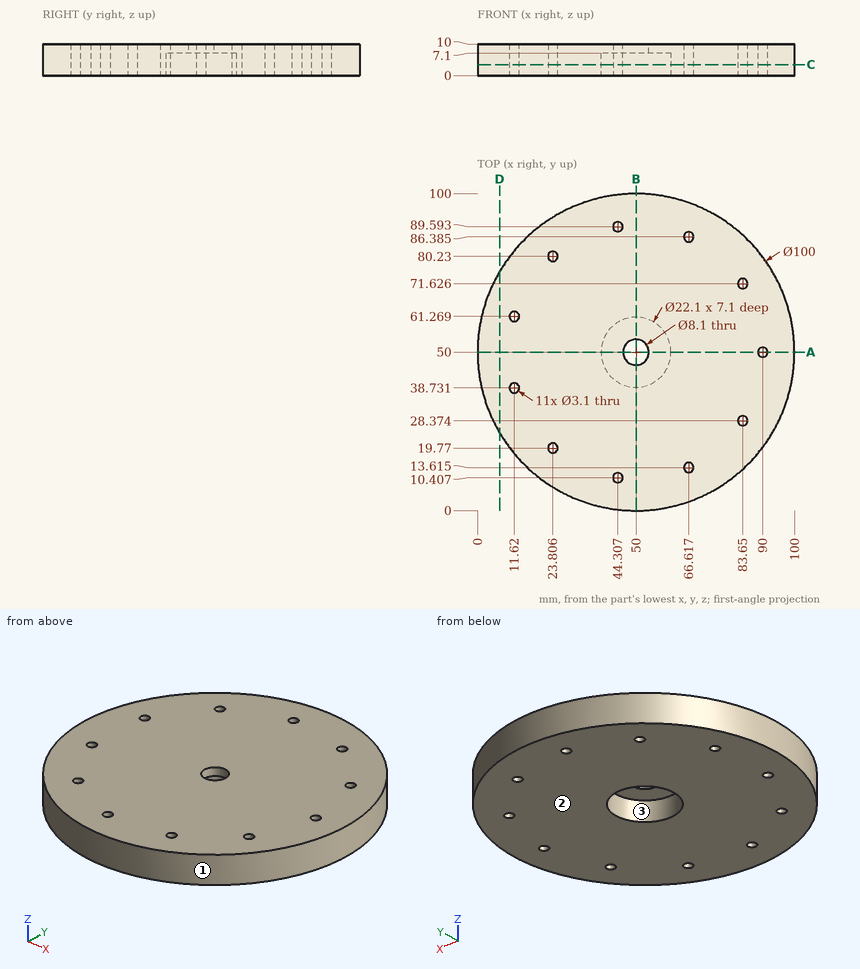
Source: three-view drawing plus pictorial views. Frame: mm from the lowest corner of the part. Round coordinates to 2 decimals unless told otherwise and drop trailing zeros. Order: outer loops, then holes, each group sorted by start corner. A loop starts at its lowest first (then second) coordinate and runs counter-clockwise, first axis right, second up. Notation, with made-up numbers: (66.5, 28) - (70.5, 28) arc R13 ccw to (70.5, 36) - close; hole circle Ø2 at (-18.75, 20.5). An arc over 180 degrees is marked (long way). Write each question's results on one line, items separated by ' | '.
Item 1: Section A-A, the plane y = 50. Return the cut outline in (x, z).
Completed:
outline: (0, 0) - (38.95, 0) - (38.95, 7.1) - (45.95, 7.1) - (45.95, 10) - (0, 10) - close; (54.05, 7.1) - (61.05, 7.1) - (61.05, 0) - (88.45, 0) - (88.45, 10) - (54.05, 10) - close; (91.55, 0) - (100, 0) - (100, 10) - (91.55, 10) - close
Item 2: Material intervals for line 1 along Y through (x, z) = (50, 7.9); line 2 along X through (y, z) = (14.5, 9) (1 decimal); line 3 along Y through (x, z) = (49, 1.25) (1 decimal), sorted ascending. Write a range as [from, to].
Completed:
line 1: [0, 45.95], [54.05, 100] | line 2: [14.8, 65.3], [67.9, 85.2] | line 3: [0, 39], [61, 100]
Item 3: Section B-B, the plane x = 50. Return the cut outline in (y, z).
Completed:
outline: (0, 0) - (38.95, 0) - (38.95, 7.1) - (45.95, 7.1) - (45.95, 10) - (0, 10) - close; (54.05, 7.1) - (61.05, 7.1) - (61.05, 0) - (100, 0) - (100, 10) - (54.05, 10) - close
Item 4: Section C-C, the plane z = 3.5. State how many separate pieces and enclosed holes the cut face has, and give its area (3 significant figures).
Completed:
separate pieces: 1 | enclosed holes: 12 | area: 7,390 mm^2
Item 5: Mould query, pull axis Y, two halves, no side actions, for the marked faces 1, 2 and 3. Classes: pulls with the +Y half, pulls with the -Y half, needs draft (parallel to the pull), parting line crosses it, or undercut.
Completed:
face 1: parting line crosses it | face 2: needs draft | face 3: undercut
Item 6: First-contact query: pin 1 Ø1.9 at (x, y) = (83.65, 71.63) entering from -Z; pin 2 Ø4 at (y, z) = (72, 4.5) entering from -X (1 decimal); pin 3 Ø2 at (y, z) = (76, 4) entering from +X; pin 4 Ø6.5 at (x, y) = (50, 54) entering from -Z. Flat tips, straight axial feed; report the tip coordinate or a pass-through.
Completed:
pin 1: through | pin 2: x = 4.2 | pin 3: x = 93.3 | pin 4: z = 7.1
Item 7: Section D-D, the plane x = 7. Return the cut outline in (y, z) (1 decimal).
Completed:
outline: (24.5, 0) - (75.5, 0) - (75.5, 10) - (24.5, 10) - close
